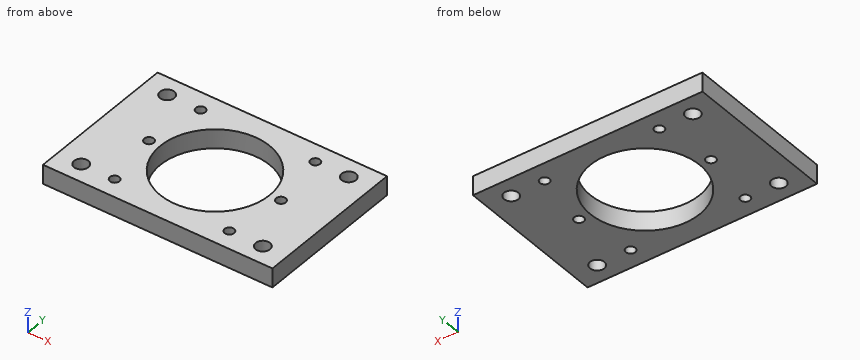
```python
from build123d import *

# Parameters (mm, degrees)
SKETCH1_W               = 76.2
SKETCH1_H               = 50.8
BOSS_EXTRUDE1_DEPTH     = 6.35
CAVITY5_OUTLINE_R       = 18.161
CAVITY5_OUTLINE_R_2     = 1.5875
CAVITY5_DEPTH           = 6.35
SKETCH3_R               = 2.38125
CUT_EXTRUDE1_DEPTH      = 92.800885072
MIRROR2_COPY_1_SKETCH_R = 2.38125
MIRROR2_COPY_1_DEPTH    = 92.800885072
SKETCH4_R               = 1.5875
CUT_EXTRUDE2_DEPTH      = 92.800885072


# Read off the part's stored shape, not the designer's step: Cavity5
with BuildPart() as part:
    # Sketch1 → Boss-Extrude1 (new body)
    with BuildSketch(Plane.XY):
        with Locations((38.1, 25.4)):
            Rectangle(SKETCH1_W, SKETCH1_H)
    extrude(amount=BOSS_EXTRUDE1_DEPTH)

    # Cavity5 outline → Cavity5 (cut)
    with BuildSketch(Plane.XY):
        with Locations((38.1, 25.4)):
            Circle(CAVITY5_OUTLINE_R)
        with Locations((16.188175065, 25.4)):
            Circle(CAVITY5_OUTLINE_R_2)
        with Locations((60.011824935, 25.4)):
            Circle(CAVITY5_OUTLINE_R_2)
    extrude(amount=CAVITY5_DEPTH, mode=Mode.SUBTRACT)

    # Sketch3 → Cut-Extrude1 (cut, through all)
    with BuildSketch(Plane(origin=(0, 0, 0), x_dir=(-1, 0, 0), z_dir=(0, 0, -1))):
        with Locations((-68.2625, 44.45)):
            Circle(SKETCH3_R)
    cut_extrude1 = extrude(amount=-CUT_EXTRUDE1_DEPTH, mode=Mode.SUBTRACT)

    # Mirror1: Cut-Extrude1 across plane
    add(cut_extrude1.mirror(Plane(origin=(38.1, 0, 0), x_dir=(0, 0, 1), z_dir=(1, 0, 0))), mode=Mode.SUBTRACT)

    # Mirror2: Cut-Extrude1 across plane
    add(cut_extrude1.mirror(Plane.ZX.offset(25.4)), mode=Mode.SUBTRACT)

    # Mirror2 copy 1 sketch → Mirror2 copy 1 (cut, through all)
    with BuildSketch(Plane(origin=(76.2, 50.8, 0), x_dir=(1, 0, 0), z_dir=(0, 0, -1))):
        with Locations((-68.2625, 44.45)):
            Circle(MIRROR2_COPY_1_SKETCH_R)
    extrude(amount=-MIRROR2_COPY_1_DEPTH, mode=Mode.SUBTRACT)

    # Sketch4 → Cut-Extrude2 (cut, through all)
    with BuildSketch(Plane(origin=(0, 0, 0), x_dir=(-1, 0, 0), z_dir=(0, 0, -1))):
        with Locations((-19.05, 6.35)):
            Circle(SKETCH4_R)
        with Locations((-57.15, 6.35)):
            Circle(SKETCH4_R)
        with Locations((-19.05, 44.45)):
            Circle(SKETCH4_R)
        with Locations((-57.15, 44.45)):
            Circle(SKETCH4_R)
    extrude(amount=-CUT_EXTRUDE2_DEPTH, mode=Mode.SUBTRACT)


solid = part.part
```
Geometry check sheet. Reference: the model listing, model coordinates, mm. Coordinates: 2 decimals unless noted, no trailing zeros. Order: outer loops, then holes, each group sorted by start corner. A loop starts at its lowest first (then second) coordinate and runs counter-clockwise, first axis right, second up. Notation, with made-up numbers: (8, 14) - (62, 14) arc R12 ccw to (62, 19) - close; hole circle Ø9 at (66, 64.25). An arc over 180 degrees is marked (long way). Answer as a JSON object with one key per item and string values. Group by question number.
Item 1: Sectioned sample at A-A, the plane y = 25.4. Record the cut outline in (x, z), and give its area (3 significant figures).
Item 2: Scan lines: probe 1 along Y at (x, z) = (57.15, 2); probe 2 along Y at (x, z) = (68, 1.25); probe 3 along Y at (x, z) = (38.1, 2.75). Record each from-to range of solid material in increasing order.
Item 3: Depth check by flat-ended pin: pin 1 Ø7.5 at (x, y) = (68.26, 6.35) entering from +Z. Enter the tip coordinate at first touch or a pass-through.
Item 4: Sectioned sample at D-D, the plane y = 6.35. Record the cut outline in (x, z), and give its area (3 significant figures).
Item 5: Sectioned sample at B-B, the plane x = 19.05. Record the cut outline in (y, z).
Item 6: Sectioned sample at C-C, the plane z = 5.25. Give the number of separate pieces and of enclosed holes in the cut face, and give its area (3 significant figures).
Resolved:
{
 "1": {"outline": "(0, 0) - (14.6, 0) - (14.6, 6.35) - (0, 6.35) - close; (17.78, 0) - (19.94, 0) - (19.94, 6.35) - (17.78, 6.35) - close; (56.26, 0) - (58.42, 0) - (58.42, 6.35) - (56.26, 6.35) - close; (61.6, 0) - (76.2, 0) - (76.2, 6.35) - (61.6, 6.35) - close", "area": "213 mm^2"},
 "2": {"probe 1": "0 to 4.76, 7.94 to 42.86, 46.04 to 50.8", "probe 2": "0 to 3.98, 8.72 to 42.08, 46.82 to 50.8", "probe 3": "0 to 7.24, 43.56 to 50.8"},
 "3": {"pin 1": "z = 6.35"},
 "4": {"outline": "(0, 0) - (5.56, 0) - (5.56, 6.35) - (0, 6.35) - close; (10.32, 0) - (17.46, 0) - (17.46, 6.35) - (10.32, 6.35) - close; (20.64, 0) - (55.56, 0) - (55.56, 6.35) - (20.64, 6.35) - close; (58.74, 0) - (65.88, 0) - (65.88, 6.35) - (58.74, 6.35) - close; (70.64, 0) - (76.2, 0) - (76.2, 6.35) - (70.64, 6.35) - close", "area": "383 mm^2"},
 "5": {"outline": "(0, 0) - (4.76, 0) - (4.76, 6.35) - (0, 6.35) - close; (7.94, 0) - (42.86, 0) - (42.86, 6.35) - (7.94, 6.35) - close; (46.04, 0) - (50.8, 0) - (50.8, 6.35) - (46.04, 6.35) - close"},
 "6": {"separate pieces": "1", "enclosed holes": "11", "area": "2,720 mm^2"}
}
